Read the model definition and answer for the solid it produces. Units are mm, in the model's axes. A direction names the side the tool comes from. Coordinates: 2 decimals unless noted, no trailing zeros. Loops run counter-clockwise (first coordinate to the right, second up) from the corner with the lowest first, then second, coordinate; pieces in that order, holes last. Notation, with made-up numbers: M 17,38.25 L 30,38.25 A22 ccw 30,46.25 Z; hole C -23.5,62 d4. An arc over 180 degrees is marked long. Use one line per item in the form item = value. Start each with the question number.
1. A flat-ended cylindrical pin translates along its axis: pin 1 (0.6 mm diameter, centred on y = -0.5, z = 8, fed in from +X). Find the tip coordinate at first contact, or state that the pin passes through.
2. A tool of negligible diameter and unlimited length cuts with its end or side. For faces 1 (the flat face through (-2.5, -0.5, 8.5)), 2 (the flat face through (-1, -0.5, 8.2)), 3 (the flat face through (2.5, -0.5, 8.5)), 4 (the flat face through (-1.8, -0.5, 9.547)), from which of +Z, -Z, +X, -X, +Y, -Y can it reach the whole face along a straight path? Write none if from no direction.
3. The part is cut by section B-B (x = 1.75). Give the number of separate pieces and of enclosed holes in the cut face, plus the area to 3 significant figures.
4. Find the intervals of material crossed by probe 1 along X at (y, z) = (-0.25, 0); probe 2 along Z at (x, y) = (-1.75, -0.25); probe 3 along Z at (x, y) = (4.5, -0.3), in increasing order. Write a range as [from, to].
5. For a pull along Z with two mould halves and no side action, classify faces 5 (the flat face through (-2, -1, 7)), 6 (the flat face through (1.7, -0.5, 9.547)), 7 (the cylindrical face through (1.25, -0.49, 8.76)) as released by +Z, released by -Z, zero draft, split by the parting line, or undercut.
6. The part is cut by section A-A (y = -0.3). Give the vertices of the cut face in (x, z), plus the area to 3 significant figures.
from build123d import *

# Parameters (mm, degrees)
F0_W     = 1.5
F0_H     = 1.609648519
F0_R     = 0.5
F1_DEPTH = 1
F2_SIZE  = 0.1


with BuildPart() as f1:
    # F0 (on Front) → F1 (new body)
    with BuildSketch(Plane.XZ):
        with BuildLine():
            Line((2.5, 7.9372539332), (1, 7.9372539332))
            ThreePointArc((1, 7.9372539332), (1.7581371123, 7.8044188697), (2.5, 7.5993420768))
            Line((2.5, 7.5993420768), (2.5, 7.9372539332))
        make_face()
        with BuildLine():
            ThreePointArc((-2.5, 7.5993420768), (-1.7581371123, 7.8044188697), (-1, 7.9372539332))
            Line((-1, 7.9372539332), (-2.5, 7.9372539332))
            Line((-2.5, 7.9372539332), (-2.5, 7.5993420768))
        make_face()
        with Locations((-1.75, 8.7420781927)):
            Rectangle(F0_W, F0_H)
        with Locations((-1.75, 8.7420781927)):
            Circle(F0_R, mode=Mode.SUBTRACT)
        with Locations((1.75, 8.7420781927)):
            Rectangle(F0_W, F0_H)
        with Locations((1.75, 8.7420781927)):
            Circle(F0_R, mode=Mode.SUBTRACT)
        with BuildLine():
            ThreePointArc((8, 0), (6.4807406984, 4.6904157598), (2.5, 7.5993420768))
            Line((2.5, 7.5993420768), (2.5, 6.5383484153))
            ThreePointArc((2.5, 6.5383484153), (5.7662812973, 3.9686269666), (7, 0))
            ThreePointArc((7, 0), (-3.9686269666, -5.7662812973), (-2.5, 6.5383484153))
            Line((-2.5, 6.5383484153), (-2.5, 7.5993420768))
            ThreePointArc((-2.5, 7.5993420768), (-4.6904157598, -6.4807406984), (8, 0))
        make_face()
        with BuildLine():
            ThreePointArc((2.5, 7.5993420768), (1.7581371123, 7.8044188697), (1, 7.9372539332))
            Line((1, 7.9372539332), (1, 6.9282032303))
            ThreePointArc((1, 6.9282032303), (1.7608227322, 6.7749172176), (2.5, 6.5383484153))
            Line((2.5, 6.5383484153), (2.5, 7.5993420768))
        make_face()
        with BuildLine():
            Line((-1, 6.9282032303), (-1, 7.9372539332))
            ThreePointArc((-1, 7.9372539332), (-1.7581371123, 7.8044188697), (-2.5, 7.5993420768))
            Line((-2.5, 7.5993420768), (-2.5, 6.5383484153))
            ThreePointArc((-2.5, 6.5383484153), (-1.7608227322, 6.7749172176), (-1, 6.9282032303))
        make_face()
    extrude(amount=F1_DEPTH)

    # F2
    f2_edges = [f1.edges().sort_by_distance(p)[0] for p in [
        (-1.75, -1, 9.546902),
        (-1, -1, 8.237553),
        (-2.5, -1, 8.573122),
        (0, -1, -8),
        (2.5, -1, 8.573122),
        (1.75, -1, 9.546902),
        (1, -1, 8.237553),
        (1.75, 0, 9.546902),
        (1, -0.5, 9.546902),
        (2.5, -0.5, 9.546902),
        (-1, -0.5, 9.546902),
        (-1.75, 0, 9.546902),
        (-2.5, -0.5, 9.546902),
        (-1, 0, 8.237553),
        (1, 0, 8.237553),
        (2.5, 0, 8.573122),
        (-2.5, 0, 8.573122),
        (0, 0, -8),
    ]]
    chamfer(f2_edges, length=F2_SIZE)


solid = f1.part
Computed values:
q1.pin_1 = 2.5
q2.face_1 = +Z, -X, +Y, -Y
q2.face_2 = +Z, +Y, -Y
q2.face_3 = +Z, +X, +Y, -Y
q2.face_4 = +Z, +X, -X, +Y, -Y
q3.separate_pieces = 3
q3.enclosed_holes = 0
q3.area = 2.78 mm²
q4.probe_1 = [-8, -7], [7, 8]
q4.probe_2 = [-7.81, -6.78], [6.78, 8.24], [9.24, 9.55]
q4.probe_3 = [-6.61, -5.36], [5.36, 6.61]
q5.face_5 = zero draft
q5.face_6 = released by +Z
q5.face_7 = undercut
q6.outline = M -2.5,7.6 A8 ccw long 2.5,7.6 L 2.5,9.45 L 2.4,9.55 L 1.1,9.55 L 1,9.45 L 1,6.93 A7 cw long -1,6.93 L -1,9.45 L -1.1,9.55 L -2.4,9.55 L -2.5,9.45 Z; hole C -1.75,8.74 d1; hole C 1.75,8.74 d1
q6.area = 48.8 mm²
